Design review of the part built by this model. Coordinates are the model's own, in mm. A direction names the side the tool comes from. Coordinates: 2 decimals unless noted, no trailing zeros. Loops run counter-clockwise (first coordinate to the right, second up) from the corner with the lowest first, then second, coordinate; pieces in that order, holes last. Notation, with made-up numbers: (4, 19.5) - (28, 19.5) arc R31 cw to (28, 52.5) - close; hole circle Ø3 at (-7, -39.75). An arc over 180 degrees is marked (long way). One line per question, with ' | ' between items.
Autodesk Inventor part; units mm, degrees
ref_plane "YZ Plane" through (0, 0, 0) normal (1, 0, 0) x (0, 1, 0)
ref_plane "XZ Plane" through (0, 0, 0) normal (0, 1, 0) x (-1, 0, 0)
ref_plane "XY Plane" through (0, 0, 0) normal (0, 0, 1) x (1, 0, 0)
sketch "Sketch1" plane through (0, 0, 0) normal (1, 0, 0) x (0, 1, 0)
  line L0 (31.75, 57.15) -> (-31.75, 57.15)
  line L1 (-31.75, 57.15) -> (-31.75, -57.15)
  line L2 (-31.75, -57.15) -> (31.75, -57.15)
  line L3 (31.75, -57.15) -> (31.75, 57.15)
  point P0 (0, 0)
  point P1 (31.75, 0)
  point P2 (0, 57.15)
  dimension "d0" = 114.3
  dimension "d1" = 63.5
extrude "Extrusion1" add sketch "Sketch1" along normal blind 9.525
sketch "Sketch3" plane through (9.525, 0, 0) normal (1, 0, 0) x (0, 0, -1)
  line L0 (-53.975, 28.575) -> (53.975, 28.575)
  line L1 (53.975, 28.575) -> (53.975, -28.575)
  line L2 (53.975, -28.575) -> (-53.975, -28.575)
  line L3 (-53.975, -28.575) -> (-53.975, 28.575)
  line L4 (-47.498, 22.098) -> (47.498, 22.098)
  line L5 (47.498, 22.098) -> (47.498, -22.098)
  line L6 (47.498, -22.098) -> (-47.498, -22.098)
  line L7 (-47.498, -22.098) -> (-47.498, 22.098)
  point P0 (0, 0)
  point P1 (0, 0)
  point P2 (-53.975, 0)
  point P3 (0, 28.575)
  dimension "d8" = 57.15
  dimension "d9" = 107.95
  dimension "d14" = 6.477
extrude "Extrusion3" cut sketch "Sketch3" against normal blind 3.175
fillet "Fillet1" radius 3.175 8 edges at (7.9375, 28.575, 53.975) (7.9375, -28.575, 53.975) (7.9375, -28.575, -53.975) (7.9375, 28.575, -53.975) (7.9375, -22.098, -47.498) (7.9375, 22.098, -47.498) (7.9375, 22.098, 47.498) (7.9375, -22.098, 47.498)
properties part number "plateEnd" material "Aluminum 6061"
Q1. To check wall thickness, follow line 1 along Z through (x, y) = (8.25, -17) (3 decimals); line 2 along Y through (x, z) = (8, 32.5) (3 decimals); line 3 along X through (y, z) = (-26, -40.5). State the ranges of each line that lie inside material, in increasing order.
Returned:
line 1: z = -57.15 to -53.975, -47.498 to 47.498, 53.975 to 57.15 | line 2: y = -31.75 to -28.575, -22.098 to 22.098, 28.575 to 31.75 | line 3: x = 0 to 6.35
Q2. Take a section at B-B (y = 6). Give the boundary of the cut face in (x, z) (3 decimals), plus the area to 3 significant figures.
Returned:
outline: (0, -57.15) - (9.525, -57.15) - (9.525, -53.975) - (6.35, -53.975) - (6.35, -47.498) - (9.525, -47.498) - (9.525, 47.498) - (6.35, 47.498) - (6.35, 53.975) - (9.525, 53.975) - (9.525, 57.15) - (0, 57.15) - close | area: 1,050 mm²
Q3. Take a section at C-C (z = -11.5). Give the boundary of the cut face in (x, y) (3 decimals).
Returned:
outline: (0, -31.75) - (9.525, -31.75) - (9.525, -28.575) - (6.35, -28.575) - (6.35, -22.098) - (9.525, -22.098) - (9.525, 22.098) - (6.35, 22.098) - (6.35, 28.575) - (9.525, 28.575) - (9.525, 31.75) - (0, 31.75) - close
Q4. Draft analysis for pull direction Y (two halves, no side actions). For faces 3 (the cylindrical face through (7.92, 27.62, 53.07)), 4 (the flat face through (5, -31.75, 1)), 5 (the flat face through (9.525, 0, 1)), state which applies: +Y half, -Y half, draft (parallel to the pull), parting line (faces both ways), or undercut.
Returned:
face 3: undercut | face 4: -Y half | face 5: draft
Q5. Tool access review of faces 1 (the flat face through (8, 0, 47.498)), 2 (the flat face through (9.525, -31, 0)): name each direction out of +Z, -Z, +X, -X, +Y, -Y from which nothing blocks a thin tool from reaching the whole face with its end or side.
Returned:
face 1: +X | face 2: +Z, -Z, +X, +Y, -Y
Q6. Take a section at D-D (y = 24). Give the boundary of the cut face in (x, z) (3 decimals), plus the area to 3 significant figures.
Returned:
outline: (0, -57.15) - (9.525, -57.15) - (9.525, -53.975) - (6.35, -53.975) - (6.35, 53.975) - (9.525, 53.975) - (9.525, 57.15) - (0, 57.15) - close | area: 746 mm²
Q7. Take a section at A-A (x = 7.5). Give the boundary of the cut face in (y, z) (3 decimals).
Returned:
outline: (-31.75, -57.15) - (31.75, -57.15) - (31.75, 57.15) - (-31.75, 57.15) - close; (-22.098, -44.323) arc R3.175 ccw to (-18.923, -47.498) - (18.923, -47.498) arc R3.175 ccw to (22.098, -44.323) - (22.098, 44.323) arc R3.175 ccw to (18.923, 47.498) - (-18.923, 47.498) arc R3.175 ccw to (-22.098, 44.323) - close; hole (-28.575, -50.8) arc R3.175 ccw to (-25.4, -53.975) - (25.4, -53.975) arc R3.175 ccw to (28.575, -50.8) - (28.575, 50.8) arc R3.175 ccw to (25.4, 53.975) - (-25.4, 53.975) arc R3.175 ccw to (-28.575, 50.8) - close
